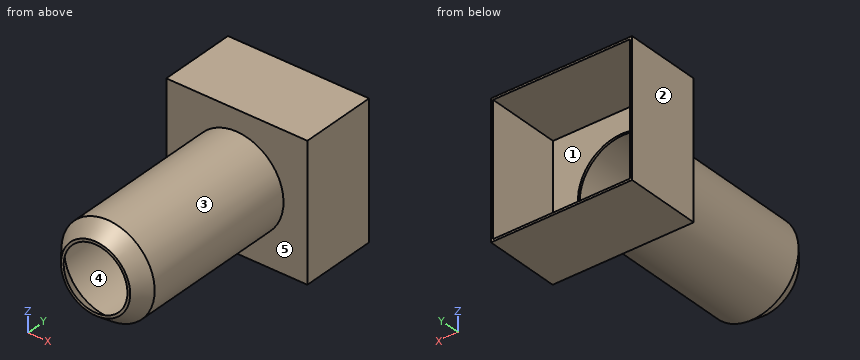
```python
from build123d import *

# Parameters (mm, degrees)
SHELL3_T                 = 0.1
BOSS_EXTRUDE1_DEPTH      = 3.1
BOSS_EXTRUDE1_DEPTH_BACK = 3.1
SKETCH1_3_W              = 3.25
SKETCH1_3_H              = 3.54
SHELL4_START             = -3
SHELL4_OUTLINE_W         = 6.3
SHELL4_OUTLINE_H         = 3.44
SHELL4_DEPTH             = 6
SKETCH2_R                = 2
CUT_EXTRUDE2_DEPTH       = 0.1


# Read off the part's stored shape, not the designer's step: Shell4
with BuildPart() as part:
    # Sketch1 → Revolve2 (revolve)
    with BuildSketch(Plane.XY, mode=Mode.PRIVATE) as revolve2_sk:
        Polygon((0, 0), (-2.05, 0), (-2.05, -7.36), (-1.469693846, -8.11), (0, -8.11), align=None)
    revolve(revolve2_sk.sketch.rotate(Axis((0, 19.440747496, 0), (0, -1, 0)), 270), axis=Axis((0, 19.440747496, 0), (0, -1, 0)))

    # Shell3
    shell3_openings = [part.faces().sort_by_distance(p)[0] for p in [
        (0, 0, 0),
        (0, -8.11, 0),
    ]]
    offset(amount=SHELL3_T, openings=shell3_openings, kind=Kind.INTERSECTION)

    # Sketch1<3> → Boss-Extrude1 (add, two sides: drawn at the far end of the back side and taken through both)
    with BuildSketch(Plane.XY.offset(-BOSS_EXTRUDE1_DEPTH_BACK)):
        Polygon((-3.25, 3.54), (-3.25, 0), (-2.05, 0), (0, 0), (0, 3.54), align=None)
        with Locations((1.625, 1.77)):
            Rectangle(SKETCH1_3_W, SKETCH1_3_H)
    extrude(amount=BOSS_EXTRUDE1_DEPTH + BOSS_EXTRUDE1_DEPTH_BACK)

    # Shell4 outline → Shell4 (cut)
    with BuildSketch(Plane.XY.offset(SHELL4_START)):
        with Locations((0, 1.82)):
            Rectangle(SHELL4_OUTLINE_W, SHELL4_OUTLINE_H)
    extrude(amount=SHELL4_DEPTH, mode=Mode.SUBTRACT)

    # Sketch2 → Cut-Extrude2 (cut)
    with BuildSketch(Plane(origin=(0, 0.1, 0), x_dir=(1, 0, 0), z_dir=(0, 1, 0))):
        with Locations(Location((0, 0, 0), (0, 0, 270))):
            Circle(SKETCH2_R)
    extrude(amount=-CUT_EXTRUDE2_DEPTH, mode=Mode.SUBTRACT)


solid = part.part
```
Check sheet for the modelled part. Datum: model origin and axes. Units: mm. Face numbers are marked on the shaded views. A direction names the side the tool comes from. Give positions to 0.01 mm unless a question says otherwise; leave off trailing zeros. Order: outer loops, then holes, each group sorted by start corner. A loop starts at its lowest first (then second) coordinate and runs counter-clockwise, first axis right, second up. Notation, with made-up numbers: (-36.5, 67) -> (-15.5, 67) arc R32 cw to (-15.5, 99) -> close; hole circle Ø7 at (-33.75, 61). An arc over 180 degrees is marked (long way). Use CSV: the item, a comma, the result in double quotes. Start each with the question number.
1) Mould release check, pull along X, two halves, no side actions. Record for the marked faces 3, 4 and 5: released by +X, released by -X, zero draft, split by the parting line, or undercut.
2) Sectioned sample at B-B, the plane x = 0. Record the boundary of the cut face in (y, z), plus the area to 3 significant figures.
3) Sectioned sample at A-A, the plane z = 0. Record the boundary of the cut face in (x, y).
4) Sectioned sample at C-C, the plane z = 2.5. Record the boundary of the cut face in (x, y), plus the area to 3 significant figures.
5) Set-up check for the marked faces 1 and 2: record each of +Z, -Z, +X, -X, +Y, -Y from which the full face is reachable in a straight line by a thin tool's end or side.
6) Material ranges on line 1 (Z direction, x = 1.75, y = -5); line 2 (Y direction, x = 1.25, z = 1.5); line 3 (Y direction, x = -1, z = 1.5), recorded low to high. Write a range as from..to.
7) Sectioned sample at D-D, the plane y = -1.25. Record the boundary of the cut face in (x, z), plus the area to 3 significant figures.
8) Go/stop test with flat-tipped pins: P1, Ø1, axis at y = -2.5, z = -2, coming from the -X side; P2, Ø3.5, axis at x = 0, z = 0, coming from the +Y side. Record where each tip stops, or that it passes through.
Recorded:
1,face 3,"split by the parting line"
1,face 4,"undercut"
1,face 5,"zero draft"
2,outline,"(-8.11, -1.6) -> (-7.39, -2.15) -> (0, -2.15) -> (0, -3.1) -> (3.54, -3.1) -> (3.54, -3) -> (0.1, -3) -> (0.1, -2) -> (0, -2) -> (0, -2.05) -> (-7.36, -2.05) -> (-8.11, -1.47) -> close; (-8.11, 1.47) -> (-7.36, 2.05) -> (0, 2.05) -> (0, 2) -> (0.1, 2) -> (0.1, 3) -> (3.54, 3) -> (3.54, 3.1) -> (0, 3.1) -> (0, 2.15) -> (-7.39, 2.15) -> (-8.11, 1.6) -> close"
2,area,"2.57 mm2"
3,outline,"(-3.25, 0) -> (-2.15, 0) -> (-2.15, -7.39) -> (-1.6, -8.11) -> (-1.47, -8.11) -> (-2.05, -7.36) -> (-2.05, 0) -> (-2, 0) -> (-2, 0.1) -> (-3.15, 0.1) -> (-3.15, 3.54) -> (-3.25, 3.54) -> close; (1.47, -8.11) -> (1.6, -8.11) -> (2.15, -7.39) -> (2.15, 0) -> (3.25, 0) -> (3.25, 3.54) -> (3.15, 3.54) -> (3.15, 0.1) -> (2, 0.1) -> (2, 0) -> (2.05, 0) -> (2.05, -7.36) -> close"
4,outline,"(-3.25, 0) -> (3.25, 0) -> (3.25, 3.54) -> (3.15, 3.54) -> (3.15, 0.1) -> (-3.15, 0.1) -> (-3.15, 3.54) -> (-3.25, 3.54) -> close"
4,area,"1.34 mm2"
5,face 1,"+Y"
5,face 2,"+Z, -Z, -X, +Y, -Y"
6,line 1,"-1.25..-1.07, 1.07..1.25"
6,line 2,"-7.65..-7.49"
6,line 3,"-7.84..-7.68"
7,outline,"circle Ø4.3 at (0, 0); hole circle Ø4.1 at (0, 0)"
7,area,"1.32 mm2"
8,P1,"x = -1.54"
8,P2,"y = -7.75"
